Build history of the part. All positions in model axes, mm. Face numbers are marked on the shaded views. A direction names the side the tool comes from. Give positions to 0.01 mm unless a question says otherwise; leave off trailing zeros. Loops run counter-clockwise (first coordinate to the right, second up) from the corner with the lowest first, then second, coordinate; pieces in that order, holes last. Notation, with made-up numbers: M -15,89 L -10,89 A28 cw -10,118 Z; hole C -23.75,-27 d11. An arc over 180 degrees is marked long. Answer in a Markdown table with one row per item. Add a question column.
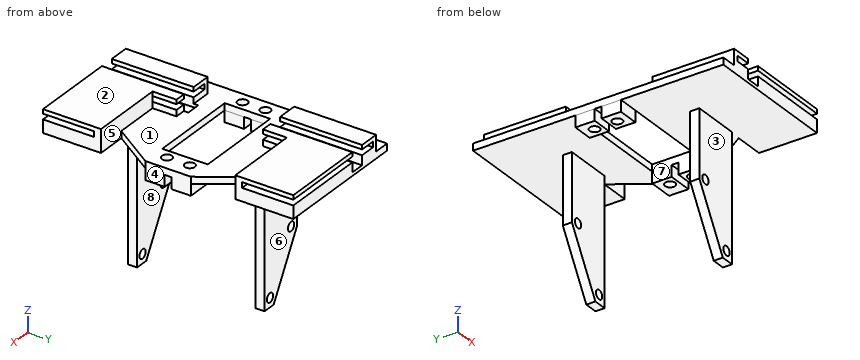
```python
from build123d import *
from build123d.topology import SkipClean

# Parameters (mm, degrees)
SKETCH_1_R               = 2.2
EXTRUDE_1_DEPTH          = 1.5
EXTRUDE_START            = -1.5
EXTRUDE_2_DEPTH          = 10
SKETCH_2_W               = 6.3
SKETCH_2_H               = 7
CUT_EXTRUDE_1_DEPTH      = 80
CUT_EXTRUDE_START        = -2
SKETCH_3_W               = 2.4
SKETCH_3_H               = 19
CUT_EXTRUDE_2_DEPTH      = 80
EXTRUDE_3_DEPTH          = 10
SKETCH_4_W               = 17.75
SKETCH_4_H               = 2.4
CUT_EXTRUDE_3_DEPTH      = 12.5
CUT_EXTRUDE_START_2      = -90
SKETCH_4_2_W             = 17.75
SKETCH_4_2_H             = 2.4
CUT_EXTRUDE_4_DEPTH      = 12.5
EXTRUDE_START_2          = -15
SKETCH_6_R               = 2
EXTRUDE_4_DEPTH          = 4
EXTRUDE_START_3          = -71
SKETCH_6_2_R             = 2
EXTRUDE_5_DEPTH          = 4
CUT_EXTRUDE_START_3      = 60
SKETCH_7_W               = 6.95
SKETCH_7_H               = 2.4
CUT_EXTRUDE_5_DEPTH      = 90
SKETCH_9_W               = 6.3
SKETCH_9_H               = 1.5
CUT_EXTRUDE_7_DEPTH      = 23
SKETCH_10_W              = 6.3
SKETCH_10_H              = 1.5
CUT_EXTRUDE_8_DEPTH      = 23
CUT_EXTRUDE_9_DEPTH      = 70
CUT_EXTRUDE_9_DEPTH_BACK = 30
SKETCH_11_W              = 2.75
SKETCH_11_H              = 2.4
EXTRUDE_6_DEPTH          = 20
EXTRUDE_7_DEPTH          = 20
SKETCH_15_W              = 37.75
SKETCH_15_H              = 1.9
EXTRUDE_8_DEPTH          = 15
SKETCH_16_W              = 37.75
SKETCH_16_H              = 1.9
EXTRUDE_9_DEPTH          = 15
EXTRUDE_START_4          = 5
SKETCH_17_W              = 10.8
SKETCH_17_H              = 8.5
SKETCH_17_R              = 2.2
SKETCH_17_W_2            = 9.2
EXTRUDE_10_DEPTH         = 5


with BuildPart() as part:
    # 草图1 → 凸台-拉伸1 (new, symmetric)
    with BuildSketch(Plane.XY):
        Polygon((15.95, 38), (15.95, 19), (7, 19), (7, 40), (0, 40), (0, -40), (7, -40), (7, -19), (15.95, -19), (15.95, -38), (22.25, -38), (22.25, -19), (24.25, -19), (27, -19), (27, -29.5), (40, -29.5), (40, -40), (60, -10), (60, 10), (40, 40), (40, 29.5), (27, 29.5), (27, 19), (24.25, 19), (22.25, 19), (22.25, 38), align=None)
        with Locations((5, -5)):
            Circle(SKETCH_1_R, mode=Mode.SUBTRACT)
        with Locations((53.4, -5)):
            Circle(SKETCH_1_R, mode=Mode.SUBTRACT)
        with Locations((5, 5)):
            Circle(SKETCH_1_R, mode=Mode.SUBTRACT)
        Polygon((16, 10), (23, 10), (49.2, 10), (49.2, -10), (23, -10), (16, -10), (9.2, -10), (9.2, 10), align=None, mode=Mode.SUBTRACT)
        with Locations((53.4, 5)):
            Circle(SKETCH_1_R, mode=Mode.SUBTRACT)
    extrude(amount=EXTRUDE_1_DEPTH, both=True)

    # 草图1<3> → 凸台-拉伸2 (add)
    with BuildSketch(Plane.XY.offset(EXTRUDE_START)):
        Polygon((7, 19), (15.95, 19), (15.95, 38), (22.25, 38), (22.25, 19), (24.25, 19), (24.25, 40), (22.25, 40), (16.15, 40), (7, 40), align=None)
        Polygon((7, -19), (7, -40), (16.15, -40), (22.25, -40), (24.25, -40), (24.25, -19), (22.25, -19), (22.25, -38), (15.95, -38), (15.95, -19), align=None)
    extrude(amount=EXTRUDE_2_DEPTH)

    # 草图2 → 切除-拉伸1 (cut)
    with BuildSketch(Plane.XZ.offset(40)):
        with Locations((19.1, 5)):
            Rectangle(SKETCH_2_W, SKETCH_2_H)
    extrude(amount=-CUT_EXTRUDE_1_DEPTH, mode=Mode.SUBTRACT)

    # 草图3 → 切除-拉伸2 (cut)
    with BuildSketch(Plane.ZY.offset(-7).offset(CUT_EXTRUDE_START)):
        with Locations((5.4, -28.5)):
            Rectangle(SKETCH_3_W, SKETCH_3_H)
        with Locations((5.4, 28.5)):
            Rectangle(SKETCH_3_W, SKETCH_3_H)
    extrude(amount=-CUT_EXTRUDE_2_DEPTH, mode=Mode.SUBTRACT)

    # 草图1<4> → 凸台-拉伸3 (add)
    with BuildSketch(Plane.XY.offset(EXTRUDE_START)):
        Polygon((24.25, 45), (24.25, 19), (27, 19), (27, 29.5), (40, 29.5), (40, 45), align=None)
        Polygon((24.25, -19), (24.25, -45), (40, -45), (40, -29.5), (27, -29.5), (27, -19), align=None)
    extrude(amount=EXTRUDE_3_DEPTH)

    # 草图4 → 切除-拉伸3 (cut)
    with BuildSketch(Plane.XZ.offset(45)):
        with Locations((31.125, 5.4)):
            Rectangle(SKETCH_4_W, SKETCH_4_H)
    extrude(amount=-CUT_EXTRUDE_3_DEPTH, mode=Mode.SUBTRACT)

    # 草图4<2> → 切除-拉伸4 (cut)
    with BuildSketch(Plane.XZ.offset(45).offset(CUT_EXTRUDE_START_2)):
        with Locations((31.125, 5.4)):
            Rectangle(SKETCH_4_2_W, SKETCH_4_2_H)
    extrude(amount=CUT_EXTRUDE_4_DEPTH, mode=Mode.SUBTRACT)

    # 草图6 → 凸台-拉伸4 (add)
    with BuildSketch(Plane(origin=(0, 45, 0), x_dir=(1, 0, 0), z_dir=(0, 1, 0)).offset(EXTRUDE_START_2)):
        Polygon((21.0788144, 1.5), (42, 1.5), (42, 7.5), (42, 56.89407293), (36.129535456, 56.89407293), (21.0788144, 30.93796809), align=None)
        with Locations(Location((25, 29.5, 0), (0, 0, 270))):
            Circle(SKETCH_6_R, mode=Mode.SUBTRACT)
        with Locations(Location((38.5, 52.8826859, 0), (0, 0, 270))):
            Circle(SKETCH_6_R, mode=Mode.SUBTRACT)
    extrude(amount=-EXTRUDE_4_DEPTH)

    # 草图6<2> → 凸台-拉伸5 (add)
    with BuildSketch(Plane(origin=(0, 45, 0), x_dir=(1, 0, 0), z_dir=(0, 1, 0)).offset(EXTRUDE_START_3)):
        Polygon((21.0788144, 1.5), (42, 1.5), (42, 7.5), (42, 56.89407293), (36.129535456, 56.89407293), (21.0788144, 30.93796809), align=None)
        with Locations(Location((25, 29.5, 0), (0, 0, 270))):
            Circle(SKETCH_6_2_R, mode=Mode.SUBTRACT)
        with Locations(Location((38.5, 52.8826859, 0), (0, 0, 270))):
            Circle(SKETCH_6_2_R, mode=Mode.SUBTRACT)
    extrude(amount=-EXTRUDE_5_DEPTH)

    # 草图7 → 切除-拉伸5 (cut)
    with BuildSketch(Plane.XZ.offset(-19).offset(CUT_EXTRUDE_START_3)):
        with Locations((12.475, 5.4)):
            Rectangle(SKETCH_7_W, SKETCH_7_H)
    extrude(amount=-CUT_EXTRUDE_5_DEPTH, mode=Mode.SUBTRACT)

    # 草图9 → 切除-拉伸7 (cut)
    with BuildSketch(Plane(origin=(0, 40, 0), x_dir=(1, 0, 0), z_dir=(0, 1, 0))):
        with Locations((19.1, -0.75)):
            Rectangle(SKETCH_9_W, SKETCH_9_H)
    extrude(amount=-CUT_EXTRUDE_7_DEPTH, mode=Mode.SUBTRACT)

    # 草图10 → 切除-拉伸8 (cut)
    with BuildSketch(Plane.XZ.offset(40)):
        with Locations((19.1, 0.75)):
            Rectangle(SKETCH_10_W, SKETCH_10_H)
    extrude(amount=-CUT_EXTRUDE_8_DEPTH, mode=Mode.SUBTRACT)

    # 草图11 → 切除-拉伸9 (cut, two sides: drawn at the far end of the back side and taken through both)
    with BuildSketch(Plane.XZ.offset(-19).offset(-CUT_EXTRUDE_9_DEPTH_BACK)):
        with Locations((25.625, 5.4)):
            Rectangle(SKETCH_11_W, SKETCH_11_H)
    extrude(amount=CUT_EXTRUDE_9_DEPTH + CUT_EXTRUDE_9_DEPTH_BACK, mode=Mode.SUBTRACT)

    # 草图12 → 凸台-拉伸6 (add)
    with BuildSketch(Plane(origin=(40, 0, 0), x_dir=(0, 0, -1), z_dir=(1, 0, 0))):
        Polygon((-8.5, -45), (-8.5, -29.5), (1.5, -29.5), (1.5, -45), (-4.2, -45), (-4.2, -32.5), (-6.6, -32.5), (-6.6, -45), align=None)
    extrude(amount=EXTRUDE_6_DEPTH)

    # 草图13 → 凸台-拉伸7 (add)
    with BuildSketch(Plane(origin=(40, 0, 0), x_dir=(0, 0, -1), z_dir=(1, 0, 0))):
        Polygon((-8.5, 45), (-8.5, 29.5), (1.5, 29.5), (1.5, 45), (-4.2, 45), (-4.2, 32.5), (-6.6, 32.5), (-6.6, 45), align=None)
    extrude(amount=EXTRUDE_7_DEPTH)

    # 草图15 → 凸台-拉伸8 (add)
    with BuildSketch(Plane(origin=(0, 40, 0), x_dir=(1, 0, 0), z_dir=(0, 1, 0))):
        Polygon((0, -1.5), (7, -1.5), (7, -8.5), (15.95, -8.5), (15.95, -6.6), (9, -6.6), (9, -4.2), (15.95, -4.2), (15.95, 0), (22.25, 0), (22.25, -4.2), (60, -4.2), (60, 1.5), (0, 1.5), align=None)
        with Locations((41.125, -7.55)):
            Rectangle(SKETCH_15_W, SKETCH_15_H)
    extrude(amount=EXTRUDE_8_DEPTH)

    # 草图16 → 凸台-拉伸9 (add)
    with BuildSketch(Plane.XZ.offset(40)):
        Polygon((15.95, 8.5), (7, 8.5), (7, 1.5), (0, 1.5), (0, -1.5), (60, -1.5), (60, 4.2), (22.25, 4.2), (22.25, 0), (15.95, 0), (15.95, 4.2), (9, 4.2), (9, 6.6), (15.95, 6.6), align=None)
        with Locations((41.125, 7.55)):
            Rectangle(SKETCH_16_W, SKETCH_16_H)
    extrude(amount=EXTRUDE_9_DEPTH)

    # 草图17 → 凸台-拉伸10 (add)
    # profile 1 of 4: a face of its own
    with SkipClean():  # the faces are left unmerged after this step: merging them gives an invalid solid
        with BuildSketch(Plane(origin=(0, 0, -1.5), x_dir=(-1, 0, 0), z_dir=(0, 0, -1)).offset(EXTRUDE_START_4)):
            with Locations((-54.6, -5.75)):
                Rectangle(SKETCH_17_W, SKETCH_17_H)
            with Locations((-53.4, -5)):
                Circle(SKETCH_17_R, mode=Mode.SUBTRACT)
        # profile 2 of 4: a face of its own
        with BuildSketch(Plane(origin=(0, 0, -1.5), x_dir=(-1, 0, 0), z_dir=(0, 0, -1)).offset(EXTRUDE_START_4)):
            with Locations((-54.6, 5.75)):
                Rectangle(SKETCH_17_W, SKETCH_17_H)
            with Locations((-53.4, 5)):
                Circle(SKETCH_17_R, mode=Mode.SUBTRACT)
        # profile 3 of 4: a face of its own
        with BuildSketch(Plane(origin=(0, 0, -1.5), x_dir=(-1, 0, 0), z_dir=(0, 0, -1)).offset(EXTRUDE_START_4)):
            with Locations((-4.6, -5.75)):
                Rectangle(SKETCH_17_W_2, SKETCH_17_H)
            with Locations((-5, -5)):
                Circle(SKETCH_17_R, mode=Mode.SUBTRACT)
        # profile 4 of 4: a face of its own
        with BuildSketch(Plane(origin=(0, 0, -1.5), x_dir=(-1, 0, 0), z_dir=(0, 0, -1)).offset(EXTRUDE_START_4)):
            with Locations((-4.6, 5.75)):
                Rectangle(SKETCH_17_W_2, SKETCH_17_H)
            with Locations((-5, 5)):
                Circle(SKETCH_17_R, mode=Mode.SUBTRACT)
        extrude(amount=-EXTRUDE_10_DEPTH)


solid = part.part
```
(1) Slice it at C-C, the plane x = 18.5. Give the cut face in (y, z), then the cut area to 3 significant figures.
(2) Pull direction Y, two halves, no side cores. Call the marked faces 1, 2 and 3: +Y half, -Y half, draft (parallel to the pull), parting line (faces both ways), or undercut.
(3) Slice it at B-B, the plane z = -25.5. Give the cut face in (x, y).
(4) Tool access for the marked faces 4, 5, 6, 7 and 8: list every direction of +Z, -Z, +X, -X, +Y, -Y with a clear straight run to the whole face (end or side of a thin tool).
(5) Pin check, flat tips, straight feed: pin 1 (0.9 mm diameter, centred on x = 2.5, y = 0, fed in from -Z); pin 2 (4.5 mm diameter, centred on y = -27, z = -17, fed in from -X); pin 3 (2.5 mm diameter, centred on x = 57, z = -4.5, fed in from -Y). Stop position of each tip, or through.
(6) Slice it at D-D, the plane y = -35.5. Give the cut face in (x, z), then the cut area to 3 significant figures.
(7) Wall check: line 1 (X direction, y = 5, z = 0.35); line 2 (Z direction, x = 57, y = 43); line 3 (Y direction, x = 22.5, z = -27). Give the ranges that are in metal, low to high.
(8) Slice it at A-A, the plane x = 11.5. Give the cut face in (y, z).
Solution:
| question | item | result |
|---|---|---|
| 1 | outline | M -55,-1.5 L -10,-1.5 L -10,1.5 L -17,1.5 L -17,0 L -55,0 Z; M 10,-1.5 L 55,-1.5 L 55,0 L 17,0 L 17,1.5 L 10,1.5 Z |
| 1 | area | 156 mm^2 |
| 2 | face 1 | undercut |
| 2 | face 2 | draft |
| 2 | face 3 | -Y half |
| 3 | outline | M 21.08,-30 L 42,-30 L 42,-26 L 21.08,-26 Z; M 21.08,26 L 42,26 L 42,30 L 21.08,30 Z |
| 4 | face 4 | +Z, -Z, +X, +Y, -Y |
| 4 | face 5 | +Z, +X |
| 4 | face 6 | -Z, +X, -X, +Y |
| 4 | face 7 | +Z, -Z |
| 4 | face 8 | -Z, +X, -X |
| 5 | pin 1 | z = -1.5 |
| 5 | pin 2 | x = 21.08 |
| 5 | pin 3 | y = -10 |
| 6 | outline | M 0,-1.5 L 60,-1.5 L 60,4.2 L 22.25,4.2 L 22.25,0 L 15.95,0 L 15.95,4.2 L 9,4.2 L 9,6.6 L 15.95,6.6 L 15.95,8.5 L 7,8.5 L 7,1.5 L 0,1.5 Z; M 22.25,6.6 L 60,6.6 L 60,8.5 L 22.25,8.5 Z |
| 6 | area | 390 mm^2 |
| 7 | line 1 | 0 to 2.8, 7.2 to 9.2, 49.2 to 51.2, 55.6 to 60 |
| 7 | line 2 | -1.5 to 4.2, 6.6 to 8.5 |
| 7 | line 3 | -30 to -26, 26 to 30 |
| 8 | outline | M -55,-1.5 L -10,-1.5 L -10,1.5 L -19,1.5 L -19,4.2 L -55,4.2 Z; M -55,6.6 L -19,6.6 L -19,8.5 L -55,8.5 Z; M 10,-1.5 L 55,-1.5 L 55,4.2 L 19,4.2 L 19,1.5 L 10,1.5 Z; M 19,6.6 L 55,6.6 L 55,8.5 L 19,8.5 Z |
